Model file for the job. Use its own axes, mm. A direction names the side the tool comes from. Round coordinates to 2 decimals unless told otherwise and drop trailing zeros. Order: outer loops, then holes, each group sorted by start corner. A loop starts at its lowest first (then second) coordinate and runs counter-clockwise, first axis right, second up. Notation, with made-up numbers: M -24.5,65 L 14.5,65 A19 ccw 14.5,83 Z; hole C 58.25,84 d1. An arc over 180 degrees is marked long. Return JSON: item names as keys, results as strings. Group by question number.
Item 1: Pull direction X, two halves, no side cores. Call faces 1 (the face through (-6.76, -31.38, 3.55)), 2 (the face through (-1, 43.55, 14)): pulls with the +X half, pulls with the -X half, needs draft (parallel to the pull), parting line crosses it, or undercut.
Item 2: Which spindle directions (+Z, -Z, +X, -X, +Y, -Y) get a long thin tool onto all of the face, cutting with end or side? Do faces 3 (the face through (-42, 29, 6)), 4 (the face through (-51, 9.05, 6)), 5 (the face through (-39, 0, 37)), 6 (the face through (40, 17, 6.4)). Say none if no direction does.
Item 3: Slice it at A-A on x = -8.05. Write the cut outline in (y, z).
Item 4: Probe line 1 along X through (y, z) = (-30, 3); line 2 along X through (y, z) = (-19.5, 27.5); line 3 along Y through (x, z) = (11, 25). List the from-to ranges inside material, lowest first.
Item 5: Slice it at B-B on y = -30.2. Write the cut outline in (x, z), then the cut area to 3 significant figures.
Item 6: Slice it at D-D on y = -10. Write the cut outline in (x, z), then the cut area to 3 significant figures.
Item 7: Pin check, flat tips, straight feed: pin 1 Ø6 at (y, z) = (1, 6.5) entering from -X; pin 2 Ø11 at (x, y) = (-49.5, 19.5) entering from +Z; pin 3 Ø6 at (x, y) = (22, -15.5) entering from +Z. Stop position of each tip, or through.
Item 8: Slice it at C-C on z = 3. Give the number of separate pieces and of enclosed holes in the cut face, then the cut area to 3 significant figures.
from build123d import *

# Parameters (mm, degrees)
F0_W      = 80
F0_H      = 87.1
F1_DEPTH  = 37
F2_W      = 76
F2_H      = 83.1
F3_DEPTH  = 30
F5_D      = 3.5
F6_W      = 34.5
F6_H      = 12.4
F7_DEPTH  = 22
F8_W      = 18
F8_H      = 30.5
F9_DEPTH  = 12
F10_W     = 11.415408
F10_H     = 6
F11_DEPTH = 4.60036
F12_W     = 34.5
F12_H     = 12.4
F13_DEPTH = 22
F14_W     = 18
F14_H     = 30.5
F15_DEPTH = 12
F16_W     = 11.5
F16_H     = 6
F17_DEPTH = 5
F19_W     = 22.9
F19_H     = 12.4
F20_DEPTH = 2
F18_W     = 22.9
F18_H     = 12.4
F21_DEPTH = 2


with BuildPart() as f1:
    # F0 (on Top) → F1 (new body)
    with BuildSketch(Plane.XY):
        Rectangle(F0_W, F0_H)
    extrude(amount=F1_DEPTH)

    # F2 (on face) → F3 (cut)
    with BuildSketch(Plane.XY.offset(37)):
        Rectangle(F2_W, F2_H)
    extrude(amount=-F3_DEPTH, mode=Mode.SUBTRACT)

    # F5 (through all)
    with Locations(Plane(origin=(0, 0, 0), x_dir=(1, 0, 0), z_dir=(0, 0, -1))):
        with Locations((-8.05, 30.2), (8.05, 30.2)):
            Hole(F5_D / 2)

    # F6 (on face) → F7 (join)
    with BuildSketch(Plane(origin=(-40, 0, 0), x_dir=(0, -1, 0), z_dir=(-1, 0, 0))):
        with Locations((-26.3, 6.2)):
            Rectangle(F6_W, F6_H)
    extrude(amount=F7_DEPTH)

    # F8 (on face) → F9 (cut)
    with BuildSketch(Plane.XY.offset(12.4)):
        with Locations((-51, 26.3)):
            Rectangle(F8_W, F8_H)
    extrude(amount=-F9_DEPTH, mode=Mode.SUBTRACT)

    # F10 (on face) → F11 (cut)
    with BuildSketch(Plane(origin=(-42, 0, 0), x_dir=(0, -1, 0), z_dir=(-1, 0, 0))):
        with Locations((-16.757704, 3.4)):
            Rectangle(F10_W, F10_H)
    extrude(amount=-F11_DEPTH, mode=Mode.SUBTRACT)

    # F12 (on face) → F13 (join)
    with BuildSketch(Plane.YZ.offset(40)):
        with Locations((26.3, 6.2)):
            Rectangle(F12_W, F12_H)
    extrude(amount=F13_DEPTH)

    # F14 (on face) → F15 (cut)
    with BuildSketch(Plane.XY.offset(12.4)):
        with Locations((51, 26.3)):
            Rectangle(F14_W, F14_H)
    extrude(amount=-F15_DEPTH, mode=Mode.SUBTRACT)

    # F16 (on face) → F17 (cut)
    with BuildSketch(Plane.YZ.offset(42)):
        with Locations((16.8, 3.4)):
            Rectangle(F16_W, F16_H)
    extrude(amount=-F17_DEPTH, mode=Mode.SUBTRACT)

    # F19 (on face) → F20 (cut)
    with BuildSketch(Plane(origin=(-62, 0, 0), x_dir=(0, -1, 0), z_dir=(-1, 0, 0))):
        with Locations((-26.3, 6.2)):
            Rectangle(F19_W, F19_H)
    extrude(amount=-F20_DEPTH, mode=Mode.SUBTRACT)

    # F18 (on face) → F21 (cut)
    with BuildSketch(Plane.YZ.offset(62)):
        with Locations((26.3, 6.2)):
            Rectangle(F18_W, F18_H)
    extrude(amount=-F21_DEPTH, mode=Mode.SUBTRACT)


solid = f1.part
Output values:
{
 "1": {"face 1": "undercut", "face 2": "needs draft"},
 "2": {"face 3": "+Z", "face 4": "+Z, -Z, -X, -Y", "face 5": "+Z, +X, -X, +Y, -Y", "face 6": "none"},
 "3": {"outline": "M -43.55,0 L -31.95,0 L -31.95,7 L -41.55,7 L -41.55,37 L -43.55,37 Z; M -28.45,0 L 43.55,0 L 43.55,37 L 41.55,37 L 41.55,7 L -28.45,7 Z"},
 "4": {"line 1": "-40 to -9.79, -6.31 to 6.31, 9.79 to 40", "line 2": "-40 to -38, 38 to 40", "line 3": "-43.55 to -41.55, 41.55 to 43.55"},
 "5": {"outline": "M -40,0 L -9.8,0 L -9.8,7 L -38,7 L -38,37 L -40,37 Z; M -6.3,0 L 6.3,0 L 6.3,7 L -6.3,7 Z; M 9.8,0 L 40,0 L 40,37 L 38,37 L 38,7 L 9.8,7 Z", "area": "631 mm²"},
 "6": {"outline": "M -40,0 L 40,0 L 40,37 L 38,37 L 38,7 L -38,7 L -38,37 L -40,37 Z", "area": "680 mm²"},
 "7": {"pin 1": "x = -40", "pin 2": "z = 0.4", "pin 3": "z = 7"},
 "8": {"separate pieces": "1", "enclosed holes": "2", "area": "7,170 mm²"}
}
